Check sheet for the modelled part. Datum: model origin and axes. Units: mm. A direction names the side the tool comes from. Give positions to 0.01 mm unless a question says otherwise; leave off trailing zeros. Order: outer loops, then holes, each group sorted by start corner. A loop starts at its lowest first (then second) coordinate and runs counter-clockwise, first axis right, second up.
from build123d import *

# Parameters (mm, degrees)
BOSS_EXTRUDE1_DEPTH = 10
CUT_EXTRUDE1_START  = 4.5
CUT_EXTRUDE1_DEPTH  = 2.5
SKETCH3_R           = 2.1
CUT_EXTRUDE2_DEPTH  = 9
CUT_EXTRUDE7_START  = 1
SKETCH4_W           = 11.6
SKETCH4_H           = 12
SKETCH4_R           = 3.3
CUT_EXTRUDE7_DEPTH  = 2


with BuildPart() as part:
    # Sketch1 → Boss-Extrude1 (new body)
    with BuildSketch(Plane(origin=(0, 0, 0), x_dir=(1, 0, 0), z_dir=(0, 1, 0))):
        Polygon((4.8, 0), (0, 0), (-4.8, 0), (-4.8, -8), (4.8, -8), align=None)
    extrude(amount=BOSS_EXTRUDE1_DEPTH)

    # Sketch2 → Cut-Extrude1 (cut)
    with BuildSketch(Plane.XY.offset(CUT_EXTRUDE1_START)):
        Polygon((3.290896534, 10), (3.290896534, 5), (1.645448267, 7.85), (-1.645448267, 7.85), (-3.290896534, 5), (-3.290896534, 10), align=None)
        Polygon((-1.645448267, 2.15), (1.645448267, 2.15), (3.290896534, 5), (1.645448267, 7.85), (-1.645448267, 7.85), (-3.290896534, 5), align=None)
    extrude(amount=CUT_EXTRUDE1_DEPTH, mode=Mode.SUBTRACT)

    # Sketch3 → Cut-Extrude2 (cut, through all)
    with BuildSketch(Plane.XY):
        with Locations((0, 5)):
            Circle(SKETCH3_R)
        Polygon((0, 7.85), (2, 7.85), (2, 10), (-2, 10), (-2, 7.85), align=None)
    extrude(amount=CUT_EXTRUDE2_DEPTH, mode=Mode.SUBTRACT)

    # Sketch4 → Cut-Extrude7 (cut)
    with BuildSketch(Plane.XY.offset(CUT_EXTRUDE7_START)):
        with Locations((0, 5)):
            Rectangle(SKETCH4_W, SKETCH4_H)
        with Locations((0, 5)):
            Circle(SKETCH4_R, mode=Mode.SUBTRACT)
    extrude(amount=CUT_EXTRUDE7_DEPTH, mode=Mode.SUBTRACT)


solid = part.part
1) Draft check along X on faces 4 (the face through (-4.8, 4.9, 0.5)), 5 (the face through (2, 9, 4)), 6 (the face through (0, 0, 5)), 7 (the face through (4.8, 4.9, 0.5)). Enter one of: +X half, -X half, draft (parallel to the pull), parting line (faces both ways), or undercut.
Recorded:
face 4: -X half
face 5: undercut
face 6: draft
face 7: +X half
2) Section check C-C, the plane z = 4. Record the cut outline in (x, y).
Recorded:
outline: (-4.8, 0) - (4.8, 0) - (4.8, 10) - (2, 10) - (2, 7.85) - (-2, 7.85) - (-2, 10) - (-4.8, 10) - close; hole circle Ø4.2 at (0, 5)
3) Set-up check for faces 1 (the face through (-1.1, 1.7, 3)), 2 (the face through (-1.4, 7, 4.5)), 3 (the face through (2, 8.9, 0.5)): record each of +Z, -Z, +X, -X, +Y, -Y from which the full face is reachable in a straight line by a thin tool's end or side.
Recorded:
face 1: none
face 2: +Y
face 3: +Z, -Z, +Y
4) Material ranges on L1, parallel to Z at x = 2.5, y = 7.5; L2, parallel to Y at x = 0, z = 3.55; L3, parallel to Z at x = -3.5, y = 0.75, recorded low to high.
Recorded:
L1: z = 0 to 1, 3 to 4.5, 7 to 8
L2: y = 0 to 2.9, 7.1 to 7.85
L3: z = 0 to 1, 3 to 8
5) Section check D-D, the plane x = 0. Record the cut outline in (y, z), then the cut area to 4 significant figures.
Recorded:
outline: (0, 0) - (2.9, 0) - (2.9, 4.5) - (2.15, 4.5) - (2.15, 7) - (2.9, 7) - (2.9, 8) - (0, 8) - (0, 3) - (1.7, 3) - (1.7, 1) - (0, 1) - close; (7.1, 0) - (7.85, 0) - (7.85, 4.5) - (7.1, 4.5) - close; (7.1, 7) - (7.85, 7) - (7.85, 8) - (7.1, 8) - close
area: 22.05 mm2
6) Section check B-B, the plane x = -3.5. Record the cut outline in (y, z), then the cut area to 3 significant figures.
Recorded:
outline: (0, 0) - (10, 0) - (10, 1) - (0, 1) - close; (0, 3) - (10, 3) - (10, 8) - (0, 8) - close
area: 60.0 mm2
7) Depth check by flat-ended pin: pin 1 Ø1.1 at (x, z) = (0.5, 7.5) entering from +Y. Enter the tip coordinate at first touch or a pass-through.
Recorded:
pin 1: stops at y = 7.85
8) Section check A-A, the plane y = 9. Record the cut outline in (x, z).
Recorded:
outline: (-4.8, 0) - (-2, 0) - (-2, 1) - (-4.8, 1) - close; (-4.8, 3) - (-2, 3) - (-2, 4.5) - (-3.29, 4.5) - (-3.29, 7) - (-2, 7) - (-2, 8) - (-4.8, 8) - close; (2, 0) - (4.8, 0) - (4.8, 1) - (2, 1) - close; (2, 3) - (4.8, 3) - (4.8, 8) - (2, 8) - (2, 7) - (3.29, 7) - (3.29, 4.5) - (2, 4.5) - close
